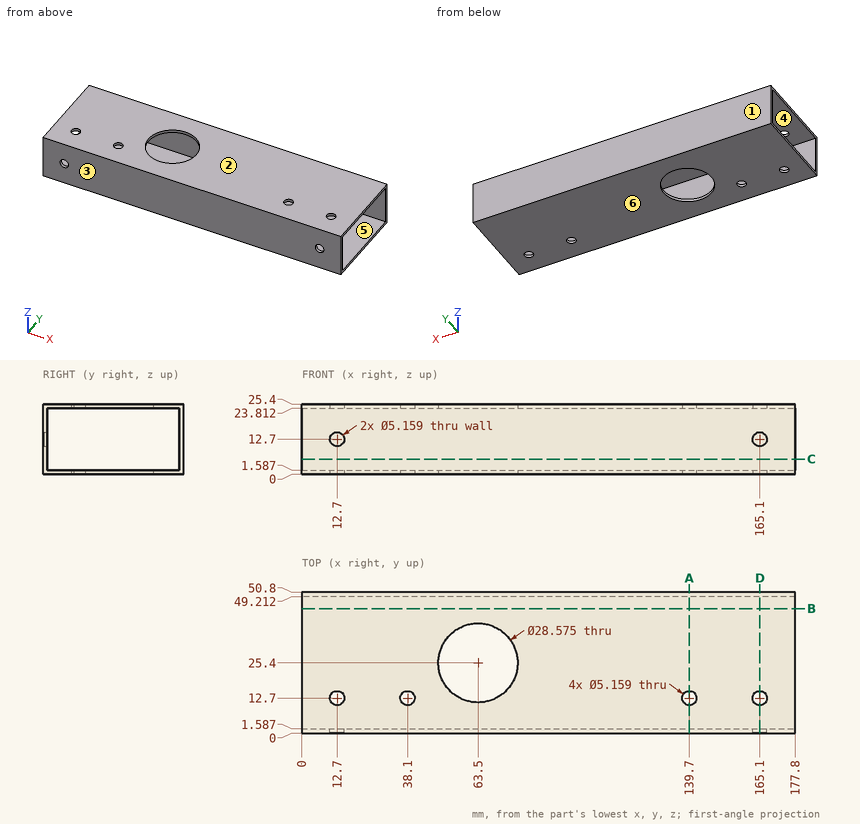
Source: three-view drawing plus pictorial views. Frame: mm from the lowest corner of the part. A direction names the side the tool comes from. Coordinates: 2 decimals unless noted, no trailing zeros. Order: outer loops, then holes, each group sorted by start corner. A loop starts at its lowest first (then second) coordinate and runs counter-clockwise, first axis right, second up. Notation, with made-up numbers: M -23,-32.75 L 24,-32.75 A28 ccw 24,-12.75 Z; hole C 5,59.25 d3. An arc over 180 degrees is marked long. Answer in a Markdown table with one row per item.
(1) Draft query along Y for the marked faces 1, 2, 3 and 4. Return one class per face: pulls with the +Y half, pulls with the -Y half, needs draft (parallel to the pull), parting line crosses it, or undercut.
Numbers:
| item | result |
|---|---|
| face 1 | pulls with the +Y half |
| face 2 | needs draft |
| face 3 | pulls with the -Y half |
| face 4 | undercut |
(2) Section query D-D, the plane x = 165.1. Output: boundary loops of the cut face in (y, z).
Numbers:
| item | result |
|---|---|
| outline | M 0,0 L 10.12,0 L 10.12,1.59 L 1.59,1.59 L 1.59,10.12 L 0,10.12 Z; M 0,15.28 L 1.59,15.28 L 1.59,23.81 L 10.12,23.81 L 10.12,25.4 L 0,25.4 Z; M 15.28,0 L 50.8,0 L 50.8,25.4 L 15.28,25.4 L 15.28,23.81 L 49.21,23.81 L 49.21,1.59 L 15.28,1.59 Z |
(3) Access query for the marked faces 5 and 6. Directions: +Z, -Z, +X, -X, +Y, -Y. A direction counts if a zero-diameter tool reaches every point of the face in a straight line with its end or side. Return the directions, or none.
Numbers:
| item | result |
|---|---|
| face 5 | +X, -X |
| face 6 | -Z, +X, -X, +Y, -Y |
(4) Section query B-B, the plane y = 45. Output: boundary loops of the cut face in (x, z).
Numbers:
| item | result |
|---|---|
| outline | M 0,0 L 177.8,0 L 177.8,1.59 L 0,1.59 Z; M 0,23.81 L 177.8,23.81 L 177.8,25.4 L 0,25.4 Z |
(5) Section query A-A, the plane x = 139.7. Output: boundary loops of the cut face in (y, z).
Numbers:
| item | result |
|---|---|
| outline | M 0,0 L 10.12,0 L 10.12,1.59 L 1.59,1.59 L 1.59,23.81 L 10.12,23.81 L 10.12,25.4 L 0,25.4 Z; M 15.28,0 L 50.8,0 L 50.8,25.4 L 15.28,25.4 L 15.28,23.81 L 49.21,23.81 L 49.21,1.59 L 15.28,1.59 Z |
(6) Section query C-C, the plane z = 5.5. Output: boundary loops of the cut face in (x, y).
Numbers:
| item | result |
|---|---|
| outline | M 0,0 L 177.8,0 L 177.8,1.59 L 0,1.59 Z; M 0,49.21 L 177.8,49.21 L 177.8,50.8 L 0,50.8 Z |
(7) Material intervals for line 1 (X direction, y = 0.85, z = 12.7); line 2 (Y direction, x = 146, z = 9.75); line 3 (Z direction, x = 116, y = 27.5), sorted ascending. Write a range as [from, to].
Numbers:
| item | result |
|---|---|
| line 1 | x = [0, 10.12], [15.28, 162.52], [167.68, 177.8] |
| line 2 | y = [0, 1.59], [49.21, 50.8] |
| line 3 | z = [0, 1.59], [23.81, 25.4] |
(8) Contact query for a flat-ended pin moving along its axis: pin 1 Ø4.5 at (x, y) = (38.1, 12.7) entering from +Z. Output: stop coordinate, or through.
Numbers:
| item | result |
|---|---|
| pin 1 | passes through |
